```python
from build123d import *

# Parameters (mm, degrees)
BOSS_EXTRUDE1_DEPTH = 6


with BuildPart() as part:
    # Sketch1 → Boss-Extrude1 (new body)
    with BuildSketch(Plane.XY):
        with BuildLine():
            Line((-55, 0), (-31.5, 0))
            ThreePointArc((-31.5, 0), (0, -31.5), (31.5, 0))
            Line((31.5, 0), (62.5, 0))
            ThreePointArc((62.5, 0), (83.75, 21.25), (105, 0))
            Line((105, 0), (105, -136))
            Line((105, -136), (60, -136))
            Line((60, -136), (60, -130))
            Line((60, -130), (-10, -130))
            Line((-10, -130), (-10, -136))
            Line((-10, -136), (-55, -136))
            Line((-55, -136), (-55, 0))
        make_face()
    extrude(amount=BOSS_EXTRUDE1_DEPTH)


solid = part.part
```
Check sheet for the modelled part. Datum: model origin and axes. Units: mm. A direction names the side the tool comes from. Coordinates: 2 decimals unless noted, no trailing zeros. Loops run counter-clockwise (first coordinate to the right, second up) from the corner with the lowest first, then second, coordinate; pieces in that order, holes last. Notation, with made-up numbers: M -6,-18 L -2,-18 A21 ccw -2,6 Z; hole C 11.5,17.5 d1. An arc over 180 degrees is marked long. Answer as a JSON object with one key per item and string values.
1. Sectioned sample at A-A on y = -8. Record the cut outline in (x, z).
Outcome:
{"outline": "M -55,0 L -30.47,0 L -30.47,6 L -55,6 Z; M 30.47,0 L 105,0 L 105,6 L 30.47,6 Z"}
2. Scan lines: L1, parallel to Y at x = 54.5, z = 5.2; L2, parallel to Y at x = -40.5, z = 1.8; L3, parallel to X at y = -0.5, z = 3.45. Record each from-to range of solid material in increasing order. Write a range as from..to.
Outcome:
{"L1": "-130..0", "L2": "-136..0", "L3": "-55..-31.5, 31.5..105"}
3. Depth check by flat-ended pin: P1, Ø2, axis at x = 32.5, z = 0.5, coming from the -Y side; P2, Ø3, axis at x = 41.5, z = 4, coming from the +Y side. Enter the tip coordinate at first touch or a pass-through.
Outcome:
{"P1": "y = -130", "P2": "y = 0"}
4. Release check for a two-part mould opening along X. For faces 1 (the flat face through (105, -67, 3)), 2 (the cylindrical face through (-0.693, -31.492, 2.958)), 3 (the flat face through (-32, -136, 3)) record: pulls with the +X half, pulls with the -X half, needs draft (parallel to the pull), parting line crosses it, or undercut.
Outcome:
{"face 1": "pulls with the +X half", "face 2": "undercut", "face 3": "needs draft"}
5. Sectioned sample at D-D on x = 0. Record the cut outline in (y, z).
Outcome:
{"outline": "M -130,0 L -31.5,0 L -31.5,6 L -130,6 Z"}
6. Sectioned sample at B-B on z = 1.95. Record the cut outline in (x, y), and give its area (3 significant figures).
Outcome:
{"outline": "M -55,-136 L -10,-136 L -10,-130 L 60,-130 L 60,-136 L 105,-136 L 105,0 A21.25 ccw 62.5,0 L 31.5,0 A31.5 cw -31.5,0 L -55,0 Z", "area": "20,500 mm²"}
7. Access from +Z, -Z, +X, -X, +Y, -Y to the whole of each face (thin tool, end or side, straight path). Record for faces 4 (the flat face through (60, -133, 3)), 5 (the flat face through (47, 0, 3)), 6 (the flat face through (-55, -69, 3)).
Outcome:
{"face 4": "+Z, -Z, -Y", "face 5": "+Z, -Z, -X, +Y", "face 6": "+Z, -Z, -X, +Y, -Y"}
8. Sectioned sample at C-C on x = -38. Record the cut outline in (y, z), and give its area (3 significant figures).
Outcome:
{"outline": "M -136,0 L 0,0 L 0,6 L -136,6 Z", "area": "816 mm²"}
